```python
from build123d import *

# Parameters (mm, degrees)
F0_W     = 40
F0_H     = 40
F1_DEPTH = 10
F2_T     = -2.54
F3_W     = 3.686494
F3_H     = 1.30985
F4_DEPTH = 4.6228


with BuildPart() as f1:
    # F0 (on Front) → F1 (new body)
    with BuildSketch(Plane.XZ):
        with Locations((20, 20)):
            Rectangle(F0_W, F0_H)
    extrude(amount=-F1_DEPTH)

    # F2
    f2_openings = [f1.faces().sort_by_distance(p)[0] for p in [
        (20, 5, 0),
    ]]
    offset(amount=F2_T, openings=f2_openings)

    # F3 (on face) → F4 (join)
    with BuildSketch(Plane(origin=(0, 0, 0), x_dir=(1, 0, 0), z_dir=(0, 0, -1))):
        with Locations((6.564244, -9.345075)):
            Rectangle(F3_W, F3_H)
    extrude(amount=F4_DEPTH)


solid = f1.part
```
For this review, take the finished solid that the model builds, in its own axes (mm). A direction names the side the tool comes from. Round coordinates to 2 decimals unless told otherwise and drop trailing zeros. Write each loop counter-clockwise with the first axis right and the second up, starting at its lowest first coordinate (ties: lowest second). Pieces come first, ordered by that corner, then holes. Notation, with made-up numbers: M 11.25,-17 L 54.25,-17 A7 cw 54.25,-12 Z; hole C -16.75,-7.5 d4. An arc over 180 degrees is marked long. One line per item, written item: value. Start each with the question number.
(1) Machinability: for faces 1 (the flat face through (0, 5, 20)), 2 (the flat face through (4.721, 9, -2)), 3 (the flat face through (37.46, 5, 18)), 4 (the flat face through (8.407, 9, -2)), 5 (the flat face through (7, 8.69, -2)), which of the approach directions +Z, -Z, +X, -X, +Y, -Y give a long, thin tool a straight path to every point of the face, cutting with its end or side? Answer none if there is none.
(2) We need section D-D (y = 1.5). Give the boundary of the cut face in (x, z).
(3) We need section A-A (z = 24). Give the boundary of the cut face in (x, y), and give its area (3 significant figures).
(4) We need section C-C (y = 5.5). Give the boundary of the cut face in (x, z), and give its area (3 significant figures).
(5) Wall thickness on line 1 (Y direction, x = 11.5, z = 16.5); line 2 (X direction, y = 6.5, z = 16.5); line 3 (Z direction, x = 22.5, y = 2.75): over which ranges is each line inside the solid? List them lowest first.
(6) Insertion check: pin 1 (2.5 mm diameter, centred on x = 27.5, y = 5, fed in from -Z); pin 2 (3 mm diameter, centred on x = 35.5, y = 6, fed in from -Z); pin 3 (1.4 mm diameter, centred on y = 9, z = -1.5, fed in from -X). Each pin has a flat end and moves straight along its axis. Give the tip position at first contact, or say it passes through.
(7) We need section B-B (x = 32.5). Give the boundary of the cut face in (y, z), and give its area (3 significant figures).
Result:
1. face 1: +Z, -Z, -X, +Y, -Y
1. face 2: -Z, -X, +Y, -Y
1. face 3: -Z
1. face 4: -Z, +X, +Y, -Y
1. face 5: -Z, +X, -X, -Y
2. outline: M 0,0 L 40,0 L 40,40 L 0,40 Z
3. outline: M 0,0 L 40,0 L 40,10 L 0,10 Z; hole M 2.54,2.54 L 37.46,2.54 L 37.46,7.46 L 2.54,7.46 Z
3. area: 228 mm²
4. outline: M 0,0 L 2.54,0 L 2.54,37.46 L 37.46,37.46 L 37.46,0 L 40,0 L 40,40 L 0,40 Z
4. area: 292 mm²
5. line 1: 0 to 2.54, 7.46 to 10
5. line 2: 0 to 2.54, 37.46 to 40
5. line 3: 37.46 to 40
6. pin 1: z = 37.46
6. pin 2: z = 0
6. pin 3: x = 4.72
7. outline: M 0,0 L 2.54,0 L 2.54,37.46 L 7.46,37.46 L 7.46,0 L 10,0 L 10,40 L 0,40 Z
7. area: 216 mm²
